Design review of the part built by this model. Coordinates are the model's own, in mm. Face numbers are marked on the shaded views. Round coordinates to 2 decimals unless told otherwise and drop trailing zeros. Order: outer loops, then holes, each group sorted by start corner. A loop starts at its lowest first (then second) coordinate and runs counter-clockwise, first axis right, second up.
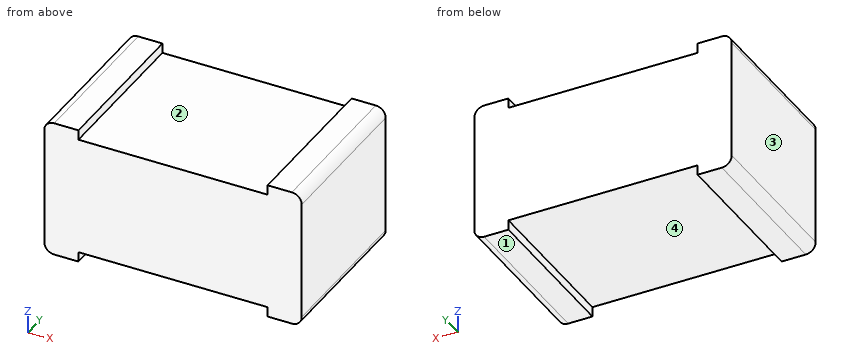
Autodesk Inventor part; units mm, degrees
ref_plane "YZ Plane" through (0, 0, 0) normal (1, 0, 0) x (0, 1, 0)
ref_plane "XZ Plane" through (0, 0, 0) normal (0, 1, 0) x (-1, 0, 0)
ref_plane "XY Plane" through (0, 0, 0) normal (0, 0, 1) x (1, 0, 0)
sketch "Sketch1" plane through (0, 0, 0) normal (0, 0, 1) x (1, 0, 0)
  line L0 (-6.5, 4) -> (6.5, 4)
  line L1 (6.5, 4) -> (6.5, -4)
  line L2 (6.5, -4) -> (-6.5, -4)
  line L3 (-6.5, -4) -> (-6.5, 4)
  point P0 (0, 0)
  point P1 (-6.5, 0)
  point P2 (0, -4)
  dimension "d0" = 8
  dimension "d1" = 13
extrude "Extrusion1" add sketch "Sketch1" along normal blind 7
sketch "Sketch2" plane through (-6.5, 4, 0) normal (0, 1, 0) x (1, 0, 0)
  line L0 (0, -7) -> (13, -7)
  line L1 (0, 0) -> (13, 0)
  line L2 (11.275, -7) -> (1.725, -7)
  line L3 (1.725, -7) -> (1.725, -6.5)
  line L4 (1.725, -6.5) -> (11.275, -6.5)
  line L5 (11.275, -6.5) -> (11.275, -7)
  line L6 (11.275, 0) -> (1.725, 0)
  line L7 (1.725, 0) -> (1.725, -0.5)
  line L8 (1.725, -0.5) -> (11.275, -0.5)
  line L9 (11.275, -0.5) -> (11.275, 0)
  line L10 (1.725, -0.05) -> (11.275, -0.05)
  line L11 (1.725, -0.3) -> (1.725, -0.05)
  line L12 (0.5, -0.3) -> (1.725, -0.3)
  line L13 (0, -0.8) -> (0.5, -0.3)
  line L14 (0, -6.2) -> (0, -0.8)
  line L15 (0.5, -6.7) -> (0, -6.2)
  line L16 (1.725, -6.7) -> (0.5, -6.7)
  line L17 (1.725, -6.7) -> (1.725, -6.75)
  line L18 (11.275, -6.75) -> (1.725, -6.75)
  line L19 (11.275, -6.7) -> (11.275, -6.75)
  line L20 (12.5, -6.7) -> (11.275, -6.7)
  line L21 (13, -6.2) -> (12.5, -6.7)
  line L22 (13, -0.8) -> (13, -6.2)
  line L23 (12.5, -0.3) -> (13, -0.8)
  line L24 (11.275, -0.3) -> (12.5, -0.3)
  line L25 (11.275, -0.3) -> (11.275, -0.05)
  point P0 (6.5, 0)
  point P1 (6.5, -7)
  point P2 (6.5, -7)
  point P3 (6.5, -0.5)
  point P4 (6.5, 0)
  dimension "d4" = 0.5
  dimension "d5" = 0.5
  dimension "d6" = 9.55
  dimension "d7" = 9.55
extrude "Extrusion2" cut sketch "Sketch2" against normal through all contours L3 L18 L5 L0 | L3 L4 L5 L18 | L7 L10 L9 L8 | L7 L1 L9 L10
fillet "Fillet1" radius 0.5 4 edges at (6.5, 0, 7) (6.5, 0, 0) (-6.5, 0, 0) (-6.5, 0, 7)
equation "\"d7\" = d6"
properties part number "SPDT Toggle Switch Base"
1) To check wall thickness, follow line 1 along Z through (x, y) = (-2.5, 1.25); line 2 along Z through (x, y) = (6.25, 3.75). State the ranges of each line that lie inside material, in increasing order.
Results:
line 1: z = 0.5 to 6.5
line 2: z = 0.07 to 6.93
2) Take a section at A-A on y = 1.25. Give the boundary of the cut face in (x, z) (3 decimals), plus the area to 3 significant figures.
Results:
outline: (-6.5, 0.5) arc R0.5 ccw to (-6, 0) - (-4.775, 0) - (-4.775, 0.5) - (4.775, 0.5) - (4.775, 0) - (6, 0) arc R0.5 ccw to (6.5, 0.5) - (6.5, 6.5) arc R0.5 ccw to (6, 7) - (4.775, 7) - (4.775, 6.5) - (-4.775, 6.5) - (-4.775, 7) - (-6, 7) arc R0.5 ccw to (-6.5, 6.5) - close
area: 81.2 mm2
3) Take a section at B-B on x = 3. Give the boundary of the cut face in (y, z), plus the area to 3 significant figures.
Results:
outline: (-4, 0.5) - (4, 0.5) - (4, 6.5) - (-4, 6.5) - close
area: 48.0 mm2
4) Clearance check with flat-ended pins moving along their axes: P1, Ø4, axis at x = -1.5, y = 1, coming from the -Z side; P2, Ø2.5, axis at x = 1.5, y = -0.5, coming from the +Z side. State where each tip first meets the part, or that it passes through.
Results:
P1: stops at z = 0.5
P2: stops at z = 6.5
5) The part is to be moulded in two halves that separate along X. For the marked faces 1, 2, 3 and 4, say which applies: released by +X, released by -X, zero draft, split by the parting line, or undercut.
Results:
face 1: zero draft
face 2: undercut
face 3: released by -X
face 4: undercut
